from build123d import *

# Parameters (mm, degrees)
SKETCH1_R               = 38.1127
BOSS_EXTRUDE1_DEPTH     = 9.525
SKETCH2_R               = 1.651
SKETCH2_R_2             = 4.1275
SKETCH2_R_3             = 11.8745
SKETCH2_R_4             = 3.175
CUT_EXTRUDE1_DEPTH      = 10.525
SKETCH4_R               = 2.3749
CUT_EXTRUDE2_DEPTH      = 6.35
CIRPATTERN1_COUNT       = 3
SKETCH5_R               = 2.38125
CUT_EXTRUDE3_DEPTH      = 1.0000001
CUT_EXTRUDE3_DEPTH_BACK = 10.5250001


with BuildPart() as part:
    # Sketch1 → Boss-Extrude1 (new body)
    with BuildSketch(Plane(origin=(0, 0, 0), x_dir=(1, 0, 0), z_dir=(0, 1, 0))):
        Circle(SKETCH1_R)
    extrude(amount=BOSS_EXTRUDE1_DEPTH)

    # Sketch2 → Cut-Extrude1 (cut, through all)
    with BuildSketch(Plane(origin=(0, 9.525, 0), x_dir=(1, 0, 0), z_dir=(0, 1, 0))):
        with Locations((0, 29.464)):
            Circle(SKETCH2_R)
        with Locations((25.516572497, -14.732)):
            Circle(SKETCH2_R)
        with Locations((-25.516572497, -14.732)):
            Circle(SKETCH2_R)
        with Locations((0, -18.415)):
            Circle(SKETCH2_R_2)
        with Locations((-12.7, 10.16)):
            Circle(SKETCH2_R_3)
        with Locations((12.7, 10.16)):
            Circle(SKETCH2_R_3)
        with Locations((0, 20.32)):
            Circle(SKETCH2_R_4)
        Circle(SKETCH2_R_4)
    extrude(amount=-CUT_EXTRUDE1_DEPTH, mode=Mode.SUBTRACT)

    # Sketch4 → Cut-Extrude2 (cut)
    with BuildSketch(Plane(origin=(-19.05635, 0, -33.006566407), x_dir=(0, -1, 0), z_dir=(-0.5, 0, -0.866025404))):
        with Locations((-4.7625, 0)):
            Circle(SKETCH4_R)
    cut_extrude2 = extrude(amount=-CUT_EXTRUDE2_DEPTH, mode=Mode.SUBTRACT)

    # CirPattern1: Cut-Extrude2 ×3 about axis
    cirpattern1_axis = Axis((0, 0, 0), (0, 1, 0))
    for i in range(1, CIRPATTERN1_COUNT):
        add(cut_extrude2.rotate(cirpattern1_axis, i * 360 / CIRPATTERN1_COUNT), mode=Mode.SUBTRACT)

    # Sketch5 → Cut-Extrude3 (cut, two sides)
    with BuildSketch(Plane(origin=(0, 9.525, 0), x_dir=(1, 0, 0), z_dir=(0, 1, 0))) as cut_extrude3_sk:
        with Locations((-15.875, -10.16)):
            Circle(SKETCH5_R)
        with Locations((15.875, -10.16)):
            Circle(SKETCH5_R)
    extrude(amount=CUT_EXTRUDE3_DEPTH, mode=Mode.SUBTRACT)
    extrude(cut_extrude3_sk.sketch, amount=-CUT_EXTRUDE3_DEPTH_BACK, mode=Mode.SUBTRACT)


solid = part.part
The model under review builds one solid part; all positions refer to its coordinate system, in mm. A direction names the side the tool comes from. Coordinates: 2 decimals unless noted, no trailing zeros. Loops run counter-clockwise (first coordinate to the right, second up) from the corner with the lowest first, then second, coordinate; pieces in that order, holes last.
(1) Wall thickness on L1, parallel to Z at x = 0, y = 6.5 (1 decimal); L2, parallel to Z at x = -16.5, y = 1.75; L3, parallel to X at y = 2, z = -10.16: over which ranges is each line inside the solid? List them lowest first.
Determined:
L1: z = -38.1 to -31.1, -27.8 to -23.5, -17.1 to -3.2, 3.2 to 14.3, 22.5 to 38.1
L2: z = -34.36 to -21.41, 1.09 to 7.86, 12.46 to 34.36
L3: x = -36.73 to -24.57, -0.83 to 0.83, 24.57 to 36.73
(2) Consider section B-B, the plane z = 0. Give the boundary of the cut face in (x, y) (3 decimals).
Determined:
outline: (-38.113, 0) - (-18.846, 0) - (-18.846, 9.525) - (-38.113, 9.525) - close; (-6.554, 0) - (-3.175, 0) - (-3.175, 9.525) - (-6.554, 9.525) - close; (3.175, 0) - (6.554, 0) - (6.554, 9.525) - (3.175, 9.525) - close; (18.846, 0) - (38.113, 0) - (38.113, 2.388) - (31.763, 2.388) - (31.763, 7.137) - (38.113, 7.137) - (38.113, 9.525) - (18.846, 9.525) - close
(3) Draft analysis for pull direction Z (two halves, no side actions). For faces 1 (the flat face through (-1, 9.525, 8)), 2 (the cylindrical face through (-25.874, 4.829, 16.344)), 3 (the cylindrical face through (-30.245, 4.696, 23.191)), state which applies: +Z half, -Z half, draft (parallel to the pull), parting line (faces both ways), or undercut.
Determined:
face 1: draft
face 2: undercut
face 3: parting line
(4) Consider section D-D, the plane z = -10.16. Give the boundary of the cut face in (x, y) (1 decimal).
Determined:
outline: (-36.7, 0) - (-24.6, 0) - (-24.6, 9.5) - (-36.7, 9.5) - close; (-0.8, 0) - (0.8, 0) - (0.8, 9.5) - (-0.8, 9.5) - close; (24.6, 0) - (36.7, 0) - (36.7, 9.5) - (24.6, 9.5) - close
(5) Consider section A-A, the plane x = 15. Give the boundary of the cut face in (y, z) (3 decimals), plus the area to 3 significant figures.
Determined:
outline: (0, -35.037) - (9.525, -35.037) - (9.525, -21.81) - (0, -21.81) - close; (0, 1.49) - (9.525, 1.49) - (9.525, 7.945) - (0, 7.945) - close; (0, 12.375) - (9.525, 12.375) - (9.525, 35.037) - (0, 35.037) - close
area: 403 mm2
(6) Consider section C-C, the plane y = 5.25. Give the number of separate pieces and of enclosed holes in the cut face, plus the area to 3 significant figures.
Determined:
separate pieces: 1
enclosed holes: 10
area: 3,410 mm2
(7) Tool access review of faces 4 (the cylindrical face through (-0.41, 4.83, -23.47)), 5 (the flat face through (-15.853, 4.796, 27.524)), 6 (the cylindrical face through (34.982, 7.135, -0.104)): name each direction out of +Z, -Z, +X, -X, +Y, -Y from which nothing blocks a thin tool from reaching the whole face with its end or side.
Determined:
face 4: +Y, -Y
face 5: none
face 6: +X
(8) Insertion check: P1, Ø2.5, axis at y = 4.5, z = -0.5, coming from the +X side; P2, Ø1.5, axis at x = -4.5, y = 1, coming from the -Z side; P3, Ø5, axis at y = 7, z = 30, coming from the +X side. Each pin has a flat end and moves straight along its axis. Give the tip position at first contact, or say it passes through.
Determined:
P1: stops at x = 31.76
P2: stops at z = -37.93
P3: stops at x = 26.39
